```python
from build123d import *
from build123d.topology import SkipClean

# Parameters (mm, degrees)
SKETCH_3_R          = 7.5
EXTRUDE_2_DEPTH     = 11.5
SKETCH_4_R          = 10
EXTRUDE_3_DEPTH     = 13
EXTRUDE_START       = 4
SKETCH_7_R          = 7.5
EXTRUDE_4_DEPTH     = 4
SKETCH_8_R          = 10
EXTRUDE_6_DEPTH     = 13
SKETCH_10_R         = 5
CUT_EXTRUDE_1_DEPTH = 25
SKETCH_11_R         = 5
CUT_EXTRUDE_2_DEPTH = 21


with BuildPart() as part:
    # Эскиз2 → Повернуть1 (revolve)
    with BuildSketch(Plane.XY, mode=Mode.PRIVATE) as revolve_1_sk:
        with BuildLine():
            Line((0, 22.5), (0, 37.5))
            ThreePointArc((0, 37.5), (5.303300859, 35.303300859), (7.5, 30))
            Line((7.5, 30), (7.5, 22.5))
            Line((7.5, 22.5), (0, 22.5))
        make_face()
    revolve(revolve_1_sk.sketch.rotate(Axis((0, 22.5, 0), (0, 1, 0)), 90), axis=Axis((0, 22.5, 0), (0, 1, 0)))

    # Эскиз3 → Бобышка-Вытянуть2 (add)
    with SkipClean():  # the faces are left unmerged after this step: merging them gives an invalid solid
        with BuildSketch(Plane.XY):
            with Locations((0, 30)):
                Circle(SKETCH_3_R)
        extrude(amount=EXTRUDE_2_DEPTH)

    # Эскиз4 → Бобышка-Вытянуть3 (add)
    with SkipClean():  # the faces are left unmerged after this step: merging them gives an invalid solid
        with BuildSketch(Plane.XY.offset(11.5)):
            with Locations(Location((0, 30, 0), (0, 0, 180))):
                Circle(SKETCH_4_R)
        extrude(amount=EXTRUDE_3_DEPTH)

    # Эскиз7 → Бобышка-Вытянуть4 (add)
    with BuildSketch(Plane.XZ.offset(-22.5).offset(EXTRUDE_START)):
        with Locations(Location((0, 0, 0), (0, 0, 270))):
            Circle(SKETCH_7_R)
    extrude(amount=-EXTRUDE_4_DEPTH)

    # Эскиз8 → Бобышка-Вытянуть6 (add)
    with BuildSketch(Plane.XZ.offset(-18.5)):
        with Locations(Location((0, 0, 0), (0, 0, 90))):
            Circle(SKETCH_8_R)
    extrude(amount=EXTRUDE_6_DEPTH)

    # Эскиз9 → Повернуть5 (revolve)
    with BuildSketch(Plane(origin=(0, 0, 0), x_dir=(0, 0, -1), z_dir=(1, 0, 0)), mode=Mode.PRIVATE) as revolve_5_sk:
        Polygon((8.5, 1.75), (6.5, 1.75), (6.5, 2.75), (9.25, 2.75), (10, 3.5), (10, 4.75), (9.5, 4.75), (9.5, 5.5), (5, 5.5), (5, 0.75), (8.5, 0.75), align=None)
    revolve(revolve_5_sk.sketch.rotate(Axis((0, 5.5, 0), (0, -1, 0)), 180), axis=Axis((0, 5.5, 0), (0, -1, 0)))

    # Эскиз14 → Повернуть6 (revolve)
    with BuildSketch(Plane(origin=(0, 0, 0), x_dir=(0, 0, -1), z_dir=(1, 0, 0)), mode=Mode.PRIVATE) as revolve_6_sk:
        Polygon((-28.25, 21.5), (-28.25, 23.5), (-27.25, 23.5), (-27.25, 20.75), (-26.5, 20), (-25.25, 20), (-25.25, 20.5), (-24.5, 20.5), (-24.5, 25), (-29.25, 25), (-29.25, 21.5), align=None)
    revolve(revolve_6_sk.sketch.rotate(Axis((0, 30, 24.5), (0, 0, 1)), 270), axis=Axis((0, 30, 24.5), (0, 0, 1)))

    # Эскиз10 → Вырез-Вытянуть1 (cut)
    with BuildSketch(Plane.XZ.offset(-5.5)):
        with Locations(Location((0, 0, 0), (0, 0, 90))):
            Circle(SKETCH_10_R)
    extrude(amount=-CUT_EXTRUDE_1_DEPTH, mode=Mode.SUBTRACT)

    # Эскиз11 → Вырез-Вытянуть2 (cut)
    with BuildSketch(Plane.XY.offset(24.5)):
        with Locations(Location((0, 30, 0), (0, 0, 180))):
            Circle(SKETCH_11_R)
    extrude(amount=-CUT_EXTRUDE_2_DEPTH, mode=Mode.SUBTRACT)


solid = part.part
```
Geometry: final body of the model. Coordinates: model frame, mm. A direction names the side the tool comes from. Round coordinates to 2 decimals unless told otherwise and drop trailing zeros. Order: outer loops, then holes, each group sorted by start corner. A loop starts at its lowest first (then second) coordinate and runs counter-clockwise, first axis right, second up. Notation, with made-up numbers: (35, -6) - (42, -6) arc R26 cw to (42, 24) - close; hole circle Ø7 at (-13.75, 18.25). An arc over 180 degrees is marked (long way). Write item = value, one per line. Start each with the question number.
Q1. Access query for faces 1 (the flat face through (-4, 39, 25.25)), 2 (the cylindrical face through (9.76, 12.09, -2.17)), 3 (the flat face through (4, 34, 29.25)). Directions: +Z, -Z, +X, -X, +Y, -Y. A direction counts if a zero-diameter tool reaches every point of the face in a straight line with its end or side. Return the directions, or none.
Q2. Pull-direction query (X, two-part tool) for faces 4 (the flat face through (4, 5.5, 9)), 5 (the flat face through (0, 32, 3.5)), 6 (the cylindrical face through (-3.92, 37.54, 28.74)); classes: +X half, -X half, draft (parallel to the pull), parting line (faces both ways), or undercut.
Q3. Pin query (flat end, axial travel): pin 1 (4 mm diameter, centred on x = 1, y = 32, fed in from +Z); pin 2 (4 mm diameter, centred on x = -4.5, y = 6, fed in from +Z); pin 3 (4 mm diameter, centred on x = 1, z = 1, fed in from -Y). Return the tip coordinate at first contact, or that it passes through.
Q4. Cut plane A-A on z = 18. Return the cut outline in (x, y), and give its area (3 significant figures).
Q5. Ray query, line 1 (Y direction, x = 0, z = 21.5); line 2 (X direction, y = 30, z = 16.75); line 3 (Z direction, x = 5.25, y = 36.5). Return the intervals inside material, ascending. Write a range as from..to.
Outcome:
q1.face_1 = none
q1.face_2 = -Y
q1.face_3 = +Z, +X, -X, +Y, -Y
q2.face_4 = draft
q2.face_5 = undercut
q2.face_6 = parting line
q3.pin_1 = 3.5
q3.pin_2 = 9.68
q3.pin_3 = 30.5
q4.outline = circle Ø20 at (0, 30); hole circle Ø10 at (0, 30)
q4.area = 236 mm^2
q5.line_1 = 20..25, 35..40
q5.line_2 = -10..-5, 5..10
q5.line_3 = 11.5..27.25, 28.25..29.25
